Autodesk Inventor part; units mm, degrees
ref_plane "YZ Plane" through (0, 0, 0) normal (1, 0, 0) x (0, 1, 0)
ref_plane "XZ Plane" through (0, 0, 0) normal (0, 1, 0) x (-1, 0, 0)
ref_plane "XY Plane" through (0, 0, 0) normal (0, 0, 1) x (1, 0, 0)
sketch "Sketch1" plane through (0, 0, 0) normal (0, 0, 1) x (1, 0, 0)
  line L0 (1.4434, 2.5) -> (2.8868, 0)
  line L1 (2.8868, 0) -> (1.4434, -2.5)
  line L2 (1.4434, -2.5) -> (-1.4434, -2.5)
  line L3 (-1.4434, -2.5) -> (-2.8868, 0)
  line L4 (-2.8868, 0) -> (-1.4434, 2.5)
  line L5 (-1.4434, 2.5) -> (1.4434, 2.5)
  point P0 (0, 0)
  point P1 (0, 0)
  dimension "d0" = 5
extrude "Extrusion1" add sketch "Sketch1" along normal blind 30
sketch "Sketch3" plane through (0, 0, 0) normal (0, 0, -1) x (-1, 0, 0)
  line L0 (1.4434, 2.5) -> (-1.4434, 2.5)
  circle A0 centre (0, 0) radius 2.5
hole "Hole1" at (0, 0, 0) direction (0, 0, 1) diameter 2.459 end through all
chamfer "Chamfer2" distance 0.5 angle 45 1 edges at (0, -1.2295, 0)
sketch "Sketch4" plane through (0, 0, 0) normal (0, 0, -1) x (-1, 0, 0)
  circle A0 centre (0, 0) radius 1.7295
  circle A1 centre (0, 0) radius 2.5
  circle A2 centre (0, 0) radius 6
extrude "Extrusion3" cut sketch "Sketch4" against normal blind 1 draft -45 contours A2
ref_plane "Work Plane1" through (0, 0, 15) normal (0, 0, -1) x (-1, 0, 0)
mirror "Mirror2" about plane through (0, 0, 15) normal (0, 0, -1) of "Extrusion3"
sketch "Sketch5" plane through (0, 0, 30) normal (0, 0, 1) x (1, 0, 0)
  circle A0 centre (0, 0) radius 1.2295
extrude "Extrusion4" add sketch "Sketch5" along normal blind 5 and the other way blind 25
thread "Thread2"
chamfer "Chamfer4" distance 0.3 angle 45 1 edges at (-1.2295, 0, 35)
properties part number "support m3 10" material "Stainless Steel"
Design review of the part built by this model. Coordinates are the model's own, in mm. A direction names the side the tool comes from. Coordinates: 2 decimals unless noted, no trailing zeros. Order: outer loops, then holes, each group sorted by start corner. A loop starts at its lowest first (then second) coordinate and runs counter-clockwise, first axis right, second up. Notation, with made-up numbers: (57.5, 35.25) -> (67.5, 35.25) arc R13 cw to (67.5, 53.25) -> close; hole circle Ø1 at (6, 11). An arc over 180 degrees is marked (long way). Use one line per item in the form item = value. Start each with the question number.
(1) Add section B-B on z = 31. State the section outline as (x, y) points.
(2) Insertion check: pin 1 (2 mm diameter, centred on y = 2, z = 4.5, fed in from -X); pin 2 (2 mm diameter, centred on x = 0.5, y = 0, fed in from -Z). Each pin has a flat end and moves straight along its axis. Give the tip position at first contact, or say it passes through.
(3) Add section A-A on z = 6. State the section outline as (x, y) points.
(4) For faces 1 (the cylindrical face through (-0.976, 0.748, 32.317)), 2 (the flat face through (0, 0, 35)), list the 3-axis set-ups (+Z, -Z, +X, -X, +Y, -Y) from which the entire face can be reached by the end or side of a thin tool; tool diameter is ignored.
(5) The part is to be moulded in two halves that separate along Y. For faces 3 (the flat face through (0, 0, 5)), 4 (the flat face through (1, 1, 30)), 5 (the flat face through (0, 2.5, 15)), 6 (the flat face through (-2.155, -1.268, 14.79)), say which applies: +Y half, -Y half, draft (parallel to the pull), parting line (faces both ways), or undercut.
(6) For probe 1 along Y at (x, z) = (0, 3.35); probe 2 along Z at (x, y) = (0.2, -0.65); probe 3 along Z at (x, y) = (2.3, 0.75), list the stretches that pass through material, from the lowest coordinate up.
Answer block:
q1.outline = circle Ø2.46 at (0, 0)
q2.pin_1 = -2.31
q2.pin_2 = 0.23
q3.outline = (-2.89, 0) -> (-1.44, -2.5) -> (1.44, -2.5) -> (2.89, 0) -> (1.44, 2.5) -> (-1.44, 2.5) -> close
q4.face_1 = +Z
q4.face_2 = +Z, +X, -X, +Y, -Y
q5.face_3 = undercut
q5.face_4 = draft
q5.face_5 = +Y half
q5.face_6 = -Y half
q6.probe_1 = -2.5 to -1.23, 1.23 to 2.5
q6.probe_2 = 5 to 35
q6.probe_3 = 0 to 30
